Geometry check sheet. Reference: drawing and pictorial views, mm from the part's lowest x, y, z. A direction names the side the tool comes from. Round coordinates to 2 decimals unless told otherwise and drop trailing zeros. Order: outer loops, then holes, each group sorted by start corner. A loop starts at its lowest first (then second) coordinate and runs counter-clockwise, first axis right, second up. Notation, with made-up numbers: (-33.75, 63) -> (11.25, 63) arc R4 ccw to (11.25, 70) -> close; hole circle Ø2 at (-17.5, 78.5). An arc over 180 degrees is marked (long way). Return JSON: item names as keys, results as strings. Group by question number.
1) Section check A-A on x = 73. Enter the section's corners in (y, z), plus the area to 3 significant figures.
2) Section check C-C on z = 20. Enter the section's corners in (x, y), plus the area to 3 significant figures.
3) Scan lines: L1, parallel to Y at x = 13, z = 56.5; L2, parallel to Z at x = 88.5, y = 72.5; L3, parallel to X at y = 14.5, z = 89.5. Record each from-to range of solid material in increasing order.
4) Draft check along Z on the marked faces 4, 5 and 6. Enter one of: pulls with the +Z half, pulls with the -Z half, needs draft (parallel to the pull), parting line crosses it, or undercut.
5) Tool access check on the marked faces 1, 2 and 3. Record the directions out of +Z, -Z, +X, -X, +Y, -Y that give a thin tool (end or side, any length) a straight path to the whole face; none if there is none.
6) Depth check by flat-ended pin: pin 1 (12 mm diameter, centred on x = 122, z = 70.5, fed in from +Y); pin 2 (10 mm diameter, centred on x = 57.5, y = 78, fed in from +Z); pin 3 (9 mm diameter, centred on x = 27, y = 50.5, fed in from -Z). Enter the tip coordinate at first touch or a pass-through.
7) Section check B-B on z = 94.5. Enter the section's corners in (x, y), plus the area to 3 significant figures.
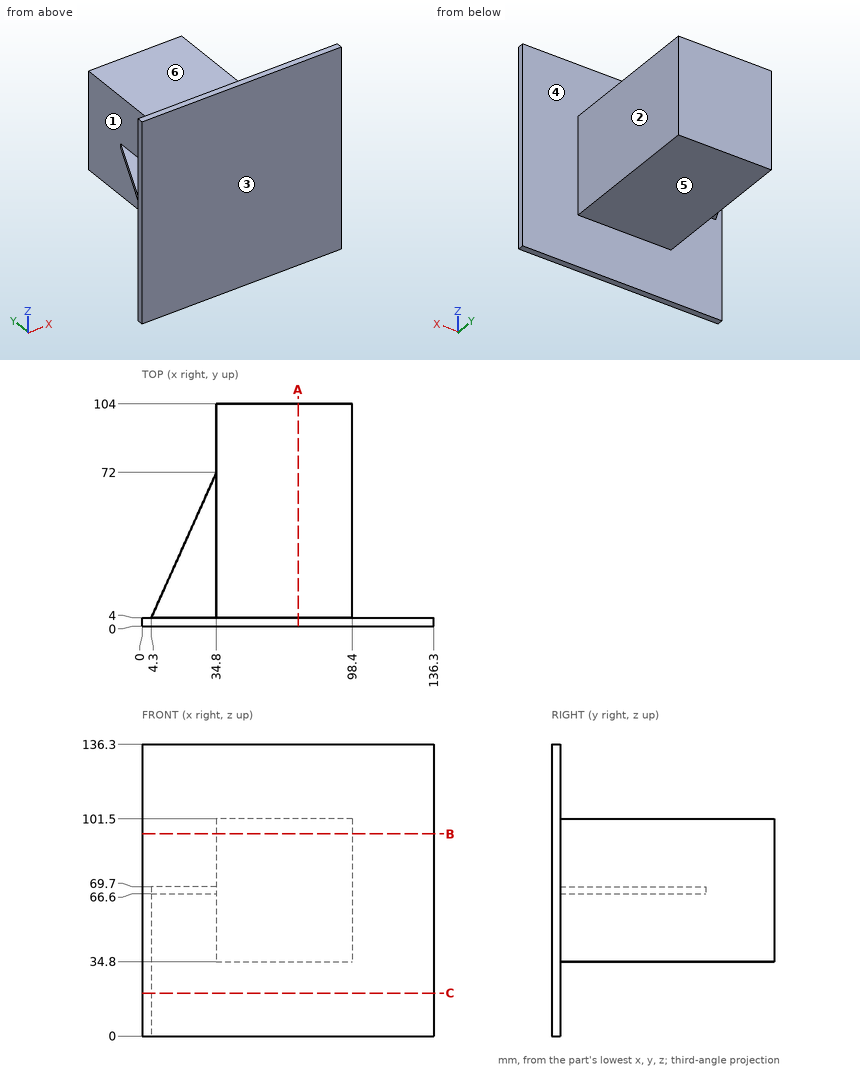
Check result:
{
 "1": {"outline": "(0, 0) -> (4, 0) -> (4, 34.8) -> (104, 34.8) -> (104, 101.5) -> (4, 101.5) -> (4, 136.3) -> (0, 136.3) -> close", "area": "7,220 mm^2"},
 "2": {"outline": "(0, 0) -> (136.3, 0) -> (136.3, 4) -> (0, 4) -> close", "area": "545 mm^2"},
 "3": {"L1": "0 to 4", "L2": "34.8 to 101.5", "L3": "34.8 to 98.4"},
 "4": {"face 4": "needs draft", "face 5": "pulls with the -Z half", "face 6": "pulls with the +Z half"},
 "5": {"face 1": "-X, +Y", "face 2": "+Z, -Z, +X, +Y", "face 3": "+Z, -Z, +X, -X, -Y"},
 "6": {"pin 1": "y = 4", "pin 2": "z = 101.5", "pin 3": "z = 66.6"},
 "7": {"outline": "(0, 0) -> (136.3, 0) -> (136.3, 4) -> (98.4, 4) -> (98.4, 104) -> (34.8, 104) -> (34.8, 4) -> (0, 4) -> close", "area": "6,910 mm^2"}
}
